Geometry: final body of the model. Coordinates: model frame, mm. A direction names the side the tool comes from. Coordinates: 2 decimals unless noted, no trailing zeros. Order: outer loops, then holes, each group sorted by start corner. A loop starts at its lowest first (then second) coordinate and runs counter-clockwise, first axis right, second up. Notation, with made-up numbers: M 48,-36 L 78,-36 A24 cw 78,-18 Z; hole C 22.5,9 d1. An arc over 180 degrees is marked long. Write item = value, one per line. Start each with the question number.
```python
from build123d import *

# Parameters (mm, degrees)
SKETCH1_R               = 65.405
BOSS_EXTRUDE1_DEPTH     = 14.732
SKETCH2_R               = 55.1688
CUT_EXTRUDE1_DEPTH      = 3.302
F_1_4_20_TAPPED_HOLE1_D = 5.1054
SKETCH6_R               = 45.72
CUT_EXTRUDE2_DEPTH      = 5.08
SKETCH7_R               = 4.826
CUT_EXTRUDE3_DEPTH      = 10.652
BOSS_EXTRUDE2_DEPTH     = 6.223


with BuildPart() as part:
    # Sketch1 → Boss-Extrude1 (new body)
    with BuildSketch(Plane.XY):
        Circle(SKETCH1_R)
    extrude(amount=BOSS_EXTRUDE1_DEPTH)

    # Sketch2 → Cut-Extrude1 (cut)
    with BuildSketch(Plane.XY.offset(14.732)):
        Circle(SKETCH2_R)
    extrude(amount=-CUT_EXTRUDE1_DEPTH, mode=Mode.SUBTRACT)

    # Sketch3 → Cut-Revolve1 (revolve, cut)
    with BuildSketch(Plane(origin=(0, 0, 0), x_dir=(0, 0, -1), z_dir=(1, 0, 0))):
        Polygon((-11.43, 34.417), (-7.747, 53.34), (-11.43, 55.1688), align=None)
    revolve(axis=Axis((0, 0, 0), (0, 0, 1)), mode=Mode.SUBTRACT)

    # 1/4-20 Tapped Hole1 (through all)
    with Locations(Plane.XY.offset(14.732)):
        with Locations((0, 60.325), (60.325, 0), (0, -60.325), (-60.325, 0)):
            Hole(F_1_4_20_TAPPED_HOLE1_D / 2)

    # Sketch6 → Cut-Extrude2 (cut)
    with BuildSketch(Plane(origin=(0, 0, 0), x_dir=(-1, 0, 0), z_dir=(0, 0, -1))):
        Circle(SKETCH6_R)
    extrude(amount=-CUT_EXTRUDE2_DEPTH, mode=Mode.SUBTRACT)

    # Sketch7 → Cut-Extrude3 (cut, through all)
    with BuildSketch(Plane(origin=(0, 0, 5.08), x_dir=(-1, 0, 0), z_dir=(0, 0, -1))):
        Circle(SKETCH7_R)
    extrude(amount=-CUT_EXTRUDE3_DEPTH, mode=Mode.SUBTRACT)

    # Sketch8 → Boss-Extrude2 (add)
    with BuildSketch(Plane(origin=(0, 0, 5.08), x_dir=(-1, 0, 0), z_dir=(0, 0, -1))):
        with BuildLine():
            Line((-13.293205934, -6.35), (-9.42734439, -6.35))
            ThreePointArc((-9.42734439, -6.35), (0, -11.3665), (9.42734439, -6.35))
            Line((9.42734439, -6.35), (13.293205934, -6.35))
            ThreePointArc((13.293205934, -6.35), (0, -14.732), (-13.293205934, -6.35))
        make_face()
        with BuildLine():
            Line((-13.293205934, 6.35), (-9.42734439, 6.35))
            ThreePointArc((-9.42734439, 6.35), (0, 11.3665), (9.42734439, 6.35))
            Line((9.42734439, 6.35), (13.293205934, 6.35))
            ThreePointArc((13.293205934, 6.35), (0, 14.732), (-13.293205934, 6.35))
        make_face()
    extrude(amount=BOSS_EXTRUDE2_DEPTH)


solid = part.part
```
Item 1: Section query B-B on y = 0. Output: boundary loops of the cut face in (x, z) (3 decimals).
Item 2: Reachability of faces 1 (the cylindrical face through (-11.96, -53.857, 13.104)), 2 (the cylindrical face through (0.156, -11.365, 2.012)), 3 (the cylindrical face through (62.875, 0.112, 7.263)) from +Z, -Z, +X, -X, +Y, -Y: full face, straight path, thin tool, end or side. Return the list, or none.
Item 3: Section query A-A on z = 3.25. Give the number of separate pieces and of enclosed holes in the cut face, and give its area (3 significant figures).
Item 4: Draft query along X for faces 4 (the flat face through (11, -6.35, 2)), 5 (the flat face through (0, 12, -1.143)), 6 (the flat face through (-11, -6.35, 2)). Return one class per face: pulls with the +X half, pulls with the -X half, needs draft (parallel to the pull), parting line crosses it, or undercut.
Item 5: First-contact query: pin 1 (3 mm diameter, centred on x = 38.5, y = -13.5, fed in from +Z); pin 2 (2 mm diameter, centred on x = -23, y = -5, fed in from -Z); pin 3 (5 mm diameter, centred on y = 46, z = 9.5, fed in from -X). Flat tips, straight axial feed; report the tip coordinate or a pass-through.
Item 6: Material intervals for probe 1 along Y at (x, z) = (0, 13) (3 decimals); probe 2 along Y at (x, z) = (0, 7.5) (3 decimals); probe 3 along X at (y, z) = (-9, 1.25), sorted ascending. Write a range as [from, to].
Ans:
q1.outline = M -65.405,0 L -62.878,0 L -62.878,14.732 L -65.405,14.732 Z; M -57.772,0 L -45.72,0 L -45.72,5.08 L -4.826,5.08 L -4.826,11.43 L -34.417,11.43 L -53.34,7.747 L -55.169,11.43 L -55.169,14.732 L -57.772,14.732 Z; M 4.826,5.08 L 45.72,5.08 L 45.72,0 L 57.772,0 L 57.772,14.732 L 55.169,14.732 L 55.169,11.43 L 53.34,7.747 L 34.417,11.43 L 4.826,11.43 Z; M 62.878,0 L 65.405,0 L 65.405,14.732 L 62.878,14.732 Z
q2.face_1 = +Z
q2.face_2 = -Z
q2.face_3 = +Z, -Z
q3.separate_pieces = 3
q3.enclosed_holes = 5
q3.area = 6,980 mm^2
q4.face_4 = undercut
q4.face_5 = needs draft
q4.face_6 = undercut
q5.pin_1 = 10.48
q5.pin_2 = 5.08
q5.pin_3 = -48.84
q6.probe_1 = [-65.405, -62.878], [-57.772, -55.169], [55.169, 57.772], [62.878, 65.405]
q6.probe_2 = [-65.405, -62.878], [-57.772, -4.826], [4.826, 57.772], [62.878, 65.405]
q6.probe_3 = [-64.78, -44.83], [-11.66, -6.94], [6.94, 11.66], [44.83, 64.78]
